Verification items for the finished model (mm, model axes). Face numbers are marked on the shaded views. Round coordinates to 2 decimals unless told otherwise and drop trailing zeros. Order: outer loops, then holes, each group sorted by start corner. A loop starts at its lowest first (then second) coordinate and runs counter-clockwise, first axis right, second up. Notation, with made-up numbers: (-39, -9) -> (-24, -9) arc R24 ccw to (-24, 20) -> close; hole circle Ø5 at (63, 50). An arc over 180 degrees is marked (long way). Put each result on its own line as item: value.
from build123d import *

# Parameters (mm, degrees)
REVOLVE1_ANGLE      = 180
BOSS_EXTRUDE1_DEPTH = 2.5
BOSS_EXTRUDE2_DEPTH = 2.5
BOSS_EXTRUDE3_DEPTH = 2.5


with BuildPart() as part:
    # Sketch1 → Revolve1 (revolve)
    with BuildSketch(Plane.XY):
        Polygon((0, 0), (45, 0), (0, 90), align=None)
    revolve(axis=Axis((0, 90, 0), (0, -1, 0)), revolution_arc=REVOLVE1_ANGLE)

    # Sketch2 → Cut-Revolve1 (revolve, cut)
    with BuildSketch(Plane(origin=(0, 0, 0), x_dir=(-1, 0, 0), z_dir=(0, 0, -1))):
        Polygon((0, 0), (0, 85), (-42.509177555, 0), align=None)
    revolve(axis=Axis((0, 0, 0), (0, 1, 0)), mode=Mode.SUBTRACT)

    # Sketch3 → Boss-Extrude1 (add)
    with BuildSketch(Plane(origin=(0, 0, 0), x_dir=(-1, 0, 0), z_dir=(0, -1, 0))):
        with BuildLine():
            Line((42.509177555, 0), (-42.509177555, 0))
            ThreePointArc((-42.509177555, 0), (0, -42.509177555), (42.509177555, 0))
        make_face()
    extrude(amount=-BOSS_EXTRUDE1_DEPTH)

    # Sketch4 → Boss-Extrude2 (add)
    with BuildSketch(Plane(origin=(0, 10, 0), x_dir=(-1, 0, 0), z_dir=(0, -1, 0))):
        with BuildLine():
            Line((-38.221336586, 0), (38.221336586, 0))
            ThreePointArc((38.221336586, 0), (0, -38.221336586), (-38.221336586, 0))
        make_face()
    extrude(amount=-BOSS_EXTRUDE2_DEPTH)

    # Sketch5 → Boss-Extrude3 (add)
    with BuildSketch(Plane(origin=(0, 20, 0), x_dir=(-1, 0, 0), z_dir=(0, -1, 0))):
        with BuildLine():
            Line((-33.5, 0), (33.5, 0))
            ThreePointArc((33.5, 0), (0, -33.5), (-33.5, 0))
        make_face()
    extrude(amount=-BOSS_EXTRUDE3_DEPTH)


solid = part.part
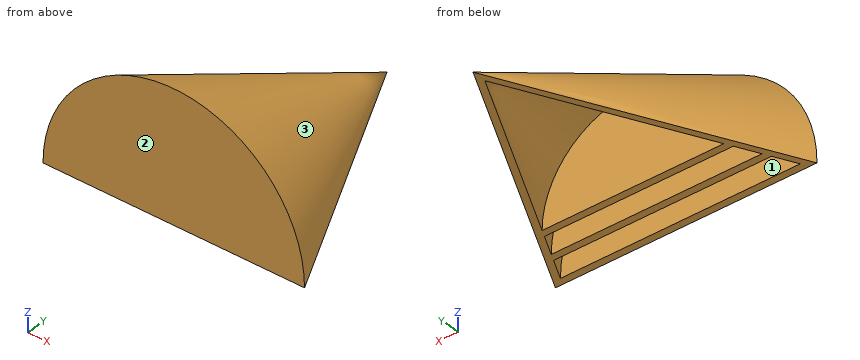
Item 1: Section check D-D on y = 40.5. Record the boundary of the cut face in (x, z).
Check sheet entries:
outline: (-24.75, 0) -> (-22.25, 0) arc R22.25 cw to (22.25, 0) -> (24.75, 0) arc R24.75 ccw to start
Item 2: Section check B-B on z = 13.5. State how many separate pieces and enclosed holes the cut face has, then the cut area to 3 significant figures.
Check sheet entries:
separate pieces: 1
enclosed holes: 3
area: 930 mm^2
Item 3: Section check A-A on x = 0. Record the boundary of the cut face in (y, z).
Check sheet entries:
outline: (0, 0) -> (2.5, 0) -> (2.5, 41.26) -> (10, 37.51) -> (10, 0) -> (12.5, 0) -> (12.5, 36.26) -> (20, 32.51) -> (20, 0) -> (22.5, 0) -> (22.5, 31.26) -> (85, 0) -> (90, 0) -> (0, 45) -> close
Item 4: Material ranges on L1, parallel to Y at x = 10.5, z = 16; L2, parallel to Y at x = -5, z = 7; L3, parallel to Y at x = -27, z = 19.5, recorded low to high. Write a range as [from, to].
Check sheet entries:
L1: y = [0, 2.5], [10, 12.5], [20, 22.5], [46.73, 51.72]
L2: y = [0, 2.5], [10, 12.5], [20, 22.5], [67.8, 72.8]
L3: y = [0, 2.5], [10, 12.5], [18.4, 23.39]
Item 5: Gauge pin test, flat ends, axial feed: pin 1 Ø4 at (x, y) = (1.5, 40) entering from -Z; pin 2 Ø3 at (x, y) = (-13.5, 18.5) entering from +Z; pin 3 Ø8 at (x, z) = (-28.5, 25.5) entering from +Y. Record the tip position at first contact, or that the pin passes through.
Check sheet entries:
pin 1: stops at z = 21.44
pin 2: stops at z = 34.1
pin 3: stops at y = 21.51
Item 6: Section check C-C on y = 82. Record the boundary of the cut face in (x, z).
Check sheet entries:
outline: (-4, 0) -> (-1.5, 0) arc R1.5 cw to (1.5, 0) -> (4, 0) arc R4 ccw to start
Item 7: Release check for a two-part mould opening along X. For the marked faces 1, 2 and 3 record: +X half, -X half, draft (parallel to the pull), parting line (faces both ways), or undercut.
Check sheet entries:
face 1: undercut
face 2: draft
face 3: parting line
